Part model, mm, in its own coordinate system. Face numbers are marked on the shaded views. A direction names the side the tool comes from. Round coordinates to 2 decimals unless told otherwise and drop trailing zeros. Loops run counter-clockwise (first coordinate to the right, second up) from the corner with the lowest first, then second, coordinate; pieces in that order, holes last.
(1) Flat gauge pins, fed straight in: pin 1 (6.5 mm diameter, centred on x = 3, z = -3, fed in from +Y); pin 2 (0.9 mm diameter, centred on x = -13.5, z = 5, fed in from +Y). Where does each tip first touch, or does it go through?
(2) Tool access for the marked faces 1, 2 and 3: list every direction of +Z, -Z, +X, -X, +Y, -Y with a clear straight run to the whole face (end or side of a thin tool).
(3) Cut at A-A on y = 13.5. List the corners of the cut face in (x, z), then the cut area to 3 significant figures.
(4) Probe probe 1 along Z at (x, y) = (-11.5, 12.25); probe 2 along X at (y, z) = (9.25, -6.5); probe 3 along Y at (x, z) = (3, 9.25). List the from-to ranges inside material, lowest first.
(5) Cut at D-D on x = 1.5. List the corners of the cut face in (y, z), then the cut area to 3 significant figures.
(6) Cut at B-B on z = -3. List the corners of the cut face in (x, y), then the cut area to 3 significant figures.
(7) Cut at C-C on y = 8.25. List the corners of the cut face in (x, z), then the cut area to 3 significant figures.
from build123d import *

# Parameters (mm, degrees)
SKETCH1_W           = 3
SKETCH1_H           = 22
BOSS_EXTRUDE3_DEPTH = 3
SKETCH1_6_W         = 25
SKETCH1_6_H         = 22
SKETCH1_6_W_2       = 5
BOSS_EXTRUDE4_DEPTH = 10
BOSS_EXTRUDE5_DEPTH = 15
SKETCH6_W           = 1.5
SKETCH6_H           = 1.5
CUT_EXTRUDE1_DEPTH  = 6


with BuildPart() as part:
    # Sketch1 → Boss-Extrude3 (new body)
    with BuildSketch(Plane(origin=(0, 0, 0), x_dir=(1, 0, 0), z_dir=(0, 1, 0))):
        with Locations((-14, 0)):
            Rectangle(SKETCH1_W, SKETCH1_H)
    extrude(amount=BOSS_EXTRUDE3_DEPTH)

    # Sketch1_6 → Boss-Extrude4 (add)
    with BuildSketch(Plane(origin=(0, 0, 0), x_dir=(1, 0, 0), z_dir=(0, 1, 0))):
        Rectangle(SKETCH1_6_W, SKETCH1_6_H)
        with Locations((-18, 0)):
            Rectangle(SKETCH1_6_W_2, SKETCH1_6_H)
    extrude(amount=BOSS_EXTRUDE4_DEPTH)

    # Sketch1_7 → Boss-Extrude5 (add)
    with BuildSketch(Plane(origin=(0, 0, 0), x_dir=(1, 0, 0), z_dir=(0, 1, 0))):
        Polygon((12.5, 11), (-12.5, 11), (-15.5, 11), (-20.5, 11), (-20.5, 15), (12.5, 15), align=None)
        Polygon((12.5, -11), (12.5, -15), (-20.5, -15), (-20.5, -11), (-15.5, -11), (-12.5, -11), align=None)
    extrude(amount=BOSS_EXTRUDE5_DEPTH)

    # Sketch6 → Cut-Extrude1 (cut)
    with BuildSketch(Plane(origin=(0, 10, 0), x_dir=(1, 0, 0), z_dir=(0, 1, 0))):
        with Locations((-16.25, 0)):
            Rectangle(SKETCH6_W, SKETCH6_H)
    extrude(amount=-CUT_EXTRUDE1_DEPTH, mode=Mode.SUBTRACT)


solid = part.part
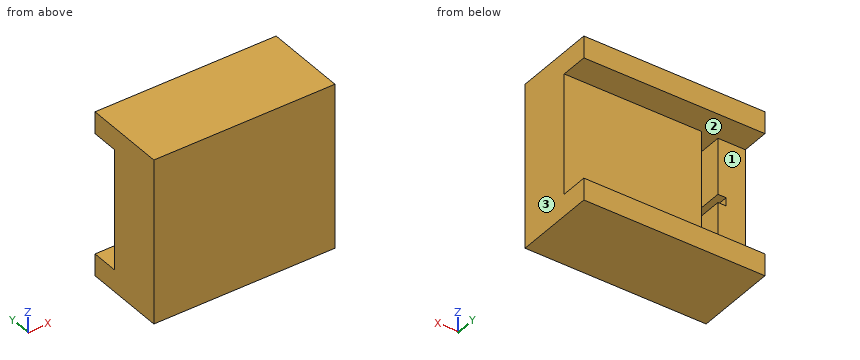
Final values:
1. pin 1: stops at y = 10
1. pin 2: stops at y = 3
2. face 1: +X, -X, +Y
2. face 2: +Y
2. face 3: +Z, -Z, +X, +Y, -Y
3. outline: (-20.5, -15) - (12.5, -15) - (12.5, -11) - (-20.5, -11) - close; (-20.5, 11) - (12.5, 11) - (12.5, 15) - (-20.5, 15) - close
3. area: 264 mm2
4. probe 1: z = -15 to -11, 11 to 15
4. probe 2: x = -20.5 to -15.5, -12.5 to 12.5
4. probe 3: y = 0 to 10
5. outline: (0, -15) - (15, -15) - (15, -11) - (10, -11) - (10, 11) - (15, 11) - (15, 15) - (0, 15) - close
5. area: 340 mm2
6. outline: (-20.5, 0) - (12.5, 0) - (12.5, 10) - (-12.5, 10) - (-12.5, 3) - (-15.5, 3) - (-15.5, 10) - (-20.5, 10) - close
6. area: 309 mm2
7. outline: (-20.5, -15) - (12.5, -15) - (12.5, 15) - (-20.5, 15) - close; hole (-17, -0.75) - (-15.5, -0.75) - (-15.5, -11) - (-12.5, -11) - (-12.5, 11) - (-15.5, 11) - (-15.5, 0.75) - (-17, 0.75) - close
7. area: 922 mm2
